from build123d import *

# Parameters (mm, degrees)
BOSS_EXTRU_1_DEPTH      = 645
ESQUISSE2_R             = 3
ENL_V_MAT_EXTRU_1_DEPTH = 955


with BuildPart() as part:
    # Esquisse1 → Boss.-Extru.1 (new body)
    with BuildSketch(Plane.XY):
        with BuildLine():
            Line((0, 0), (0, 20))
            Line((0, 20), (3, 20))
            Line((3, 20), (3, 6))
            ThreePointArc((3, 6), (3.878679656, 3.878679656), (6, 3))
            Line((6, 3), (20, 3))
            Line((20, 3), (20, 0))
            Line((20, 0), (0, 0))
        make_face()
    extrude(amount=BOSS_EXTRU_1_DEPTH)

    # Esquisse2 → Enlèv. mat.-Extru.1 (cut)
    with BuildSketch(Plane(origin=(0, 0, 0), x_dir=(-1, 0, 0), z_dir=(0, -1, 0))):
        with Locations(Location((-10, -50, 0), (0, 0, 180))):
            Circle(ESQUISSE2_R)
        with Locations(Location((-10, -595, 0), (0, 0, 180))):
            Circle(ESQUISSE2_R)
        with Locations(Location((-10, -230, 0), (0, 0, 180))):
            Circle(ESQUISSE2_R)
        with Locations(Location((-10, -415, 0), (0, 0, 180))):
            Circle(ESQUISSE2_R)
    extrude(amount=-ENL_V_MAT_EXTRU_1_DEPTH, mode=Mode.SUBTRACT)


solid = part.part
Geometry check sheet. Reference: the model listing, model coordinates, mm. A direction names the side the tool comes from. Round coordinates to 2 decimals unless told otherwise and drop trailing zeros. Loops run counter-clockwise (first coordinate to the right, second up) from the corner with the lowest first, then second, coordinate; pieces in that order, holes last.
Item 1: Cross-section at C-C on y = 11.5. Record the boundary of the cut face in (x, z), then the cut area to 4 significant figures.
Item 2: Cross-section at B-B on z = 522. Record the boundary of the cut face in (x, y), then the cut area to 3 significant figures.
Item 3: Cross-section at A-A on x = 10. Record the boundary of the cut face in (y, z).
Item 4: Gauge pin test, flat ends, axial feed: pin 1 (6 mm diameter, centred on x = 16, z = 200, fed in from +Y); pin 2 (9.5 mm diameter, centred on x = 10, z = 595, fed in from +Y); pin 3 (6 mm diameter, centred on x = 7.5, z = 119.5, fed in from +Y); pin 4 (5 mm diameter, centred on x = 10, z = 50, fed in from -Y). Record the tip position at first contact, or that the pin passes through.
Item 5: Access from +Z, -Z, +X, -X, +Y, -Y to the whole of each face (thin tool, end or side, straight path). Record for faces 1 (the flat face through (4, 3, 0)), 2 (the flat face through (3, 13, 318)).
Item 6: Thickness scan on line 1 (Z direction, x = 10, y = 1.5); line 2 (X direction, y = 1.45, z = 415); line 3 (X direction, y = 9.5, z = 166). Record the ranges inside material, lowest first.
Answer sheet:
1. outline: (0, 0) - (3, 0) - (3, 645) - (0, 645) - close
1. area: 1,935 mm2
2. outline: (0, 0) - (20, 0) - (20, 3) - (6, 3) arc R3 cw to (3, 6) - (3, 20) - (0, 20) - close
2. area: 113 mm2
3. outline: (0, 0) - (3, 0) - (3, 47) - (0, 47) - close; (0, 53) - (3, 53) - (3, 227) - (0, 227) - close; (0, 233) - (3, 233) - (3, 412) - (0, 412) - close; (0, 418) - (3, 418) - (3, 592) - (0, 592) - close; (0, 598) - (3, 598) - (3, 645) - (0, 645) - close
4. pin 1: stops at y = 3
4. pin 2: stops at y = 3.1
4. pin 3: stops at y = 3.4
4. pin 4: passes through
5. face 1: -Z, +X, -X, +Y, -Y
5. face 2: +Z, -Z, +X, +Y
6. line 1: z = 0 to 47, 53 to 227, 233 to 412, 418 to 592, 598 to 645
6. line 2: x = 0 to 7, 13 to 20
6. line 3: x = 0 to 3
